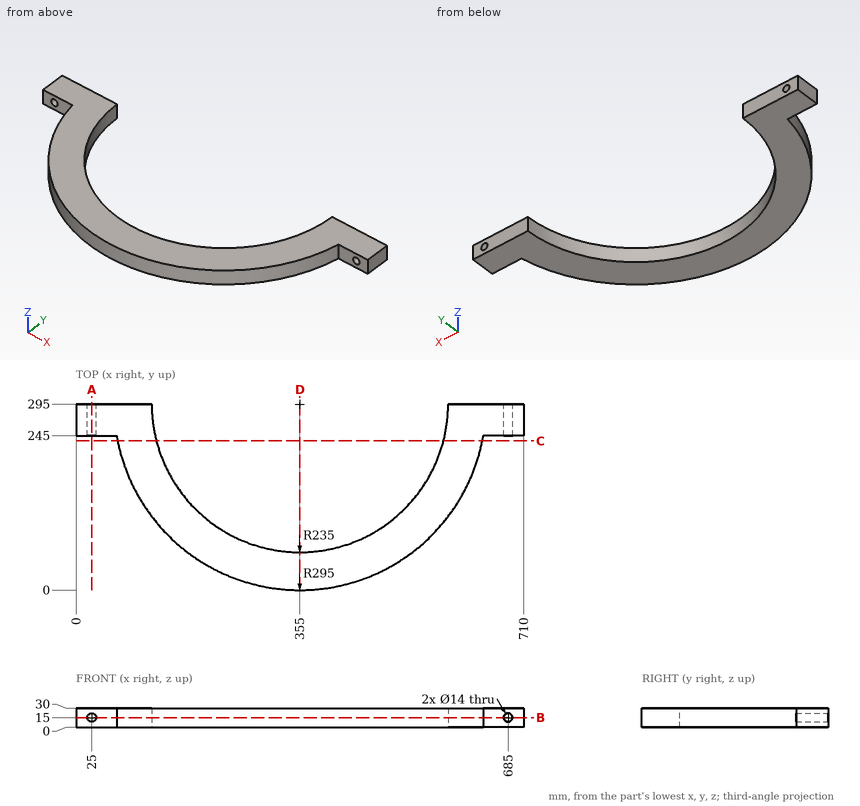
Geometry: see drawing. Coordinates: mm, zero at the bounding-box minimum. Round coordinates to 2 decimals unless told otherwise and drop trailing zeros. Write each loop counter-clockwise with the first axis right and the second up, starting at its lowest first coordinate (ties: lowest second). Pieces come first, ordered by that corner, then holes. Notation, with made-up numbers: M 82,-28 L 108,-28 A24 ccw 108,0 Z; hole C 79,73.25 d4. An arc over 180 degrees is marked long. Answer as a JSON object with one key per item and string values. Group by question number.
(1) Section query B-B on z = 15. Output: boundary loops of the cut face in (x, y).
(2) Ray query, line 1 (Z direction, x = 25, y = 272.5); line 2 (X direction, y = 260.5, z = 15); line 3 (X direction, y = 283, z = 15). Return the intervals inside material, ascending. Write a range as [from, to].
(3) Section query D-D on x = 355. Output: boundary loops of the cut face in (y, z), then the cut area to 3 significant figures.
(4) Section query A-A on x = 25. Output: boundary loops of the cut face in (y, z), then the cut area to 3 significant figures.
(5) Section query C-C on y = 236.5. Output: boundary loops of the cut face in (x, z), then the cut area to 3 significant figures.
(6) First-contact query: pin 1 (8 mm diameter, centred on y = 205, z = 6.5, fed in from +X); pin 2 (1 mm diameter, centred on x = 184.5, z = 19, fed in from -Y); pin 3 (15 mm diameter, centred on x = 27.5, z = 22, fed in from -Y). Flat tips, straight axial feed; report the tip coordinate or a pass-through.
Computed values:
{
 "1": {"outline": "M 0,245 L 18,245 L 18,295 L 0,295 Z; M 32,245 L 64.27,245 A295 ccw 645.73,245 L 678,245 L 678,295 L 590,295 A235 cw 120,295 L 32,295 Z; M 692,245 L 710,245 L 710,295 L 692,295 Z"},
 "2": {"line 1": "[0, 8], [22, 30]", "line 2": "[0, 18], [32, 122.55], [587.45, 678], [692, 710]", "line 3": "[0, 18], [32, 120.31], [589.69, 678], [692, 710]"},
 "3": {"outline": "M 0,0 L 60,0 L 60,30 L 0,30 Z", "area": "1,800 mm^2"},
 "4": {"outline": "M 245,0 L 295,0 L 295,8 L 245,8 Z; M 245,22 L 295,22 L 295,30 L 245,30 Z", "area": "800 mm^2"},
 "5": {"outline": "M 65.86,0 L 127.4,0 L 127.4,30 L 65.86,30 Z; M 582.6,0 L 644.14,0 L 644.14,30 L 582.6,30 Z", "area": "3,690 mm^2"},
 "6": {"pin 1": "x = 637.19", "pin 2": "y = 53.91", "pin 3": "y = 245"}
}
